Read the model definition and answer for the solid it produces. Units are mm, in the model's axes. Round coordinates to 2 decimals unless told otherwise and drop trailing zeros. Write each loop counter-clockwise with the first axis right and the second up, starting at its lowest first coordinate (ties: lowest second). Pieces come first, ordered by that corner, then holes. Notation, with made-up numbers: (79, -3) -> (103, -3) arc R20 ccw to (103, 33) -> close; hole circle Ø1 at (10, 46.25). An arc over 180 degrees is marked (long way). Return JSON: item names as keys, results as strings.
Solid Edge part; units mm, degrees
sketch "Sketch1" plane through (0, 0, 0) normal (0, -1, 0) x (1, 0, 0)
  line L0 (0, 0) -> (0, -2.95)
  line L1 (0, -2.95) -> (0.3349, -4.2)
  line L2 (0.3349, -4.2) -> (2.8651, -4.2)
  line L3 (2.8651, -4.2) -> (3.2, -2.95)
  line L4 (3.2, -2.95) -> (3.2, 0)
  line L5 (3.2, 0) -> (0, 0)
revolve "RevolvedProtrusion1" add sketch "Sketch1" angle 360 about axis through (3.2, 0, 0) along (-1, 0, 0)
sketch "Sketch2" plane through (0, 0, 0) normal (1, 0, 0) x (0, 1, 0)
  line L0 (14, 14) -> (-14, 14)
  line L1 (-14, 14) -> (-14, -14)
  line L2 (-14, -14) -> (14, -14)
  line L3 (14, -14) -> (14, 14)
  line L4 (2.0207, 3.5) -> (-2.0207, 3.5)
  line L5 (-2.0207, 3.5) -> (-4.0415, 0)
  line L6 (-4.0415, 0) -> (-2.0207, -3.5)
  line L7 (-2.0207, -3.5) -> (2.0207, -3.5)
  line L8 (2.0207, -3.5) -> (4.0415, 0)
  line L9 (4.0415, 0) -> (2.0207, 3.5)
extrude "ExtrudedCutout_1" cut sketch "Sketch2" against normal blind 4.2 and the other way blind 4.2
sketch "Sketch3" plane through (0, 0, 0) normal (0, 0, 1) x (1, 0, 0)
  line L0 (0, 0) -> (0, 2)
  line L1 (0, 2) -> (0.379, 1.621)
  line L2 (0.379, 1.621) -> (2.821, 1.621)
  line L3 (2.821, 1.621) -> (3.2, 2)
  line L4 (3.2, 2) -> (3.2, 0)
  line L5 (3.2, 0) -> (0, 0)
revolve "RevolvedCutout1" cut sketch "Sketch3" angle 360 about axis through (3.2, 0, 0) along (-1, 0, 0)
cosmetic_thread "Thread1"
properties part number "Hexagon nut - style 1 JIS B 1181 M4"
Item 1: Straight lines are drawn through the part: L1, parallel to Z at x = 1.9, y = 0; L2, parallel to Y at x = 0.75, z = 2; L3, parallel to Y at x = 3, z = 1.5. For each, find the intervals that lie inside material, in ascending order. Write a range as [from, to].
Worked answers:
{"L1": "z = [-3.5, -1.62], [1.62, 3.5]", "L2": "y = [-2.89, 2.89]", "L3": "y = [-3.18, -0.99], [0.99, 3.18]"}
Item 2: Section A-A (y = 0) is taken. Give the vertices of the cut face in (x, z), then the cut area to 3 significant figures.
Worked answers:
{"outline": "(0, -2.95) -> (0.15, -3.5) -> (3.05, -3.5) -> (3.2, -2.95) -> (3.2, -2) -> (2.82, -1.62) -> (0.38, -1.62) -> (0, -2) -> close; (0, 2) -> (0.38, 1.62) -> (2.82, 1.62) -> (3.2, 2) -> (3.2, 2.95) -> (3.05, 3.5) -> (0.15, 3.5) -> (0, 2.95) -> close", "area": "11.6 mm2"}
Item 3: For a pull along Z with two mould halves and no side action, classify faces 1 (the flat face through (3.2, 1, -2)), 2 (the flat face through (1.62, 3.045, 1.726)), 3 (the cylindrical face through (1.617, 0.748, -1.438)) as released by +Z, released by -Z, zero draft, split by the parting line, or undercut.
Worked answers:
{"face 1": "zero draft", "face 2": "released by +Z", "face 3": "undercut"}
Item 4: Section B-B (x = 1.5) is taken. Give the vertices of the cut face in (y, z), then the cut area to 3 significant figures.
Worked answers:
{"outline": "(-4.04, 0) -> (-2.02, -3.5) -> (2.02, -3.5) -> (4.04, 0) -> (2.02, 3.5) -> (-2.02, 3.5) -> close; hole circle Ø3.24 at (0, 0)", "area": "34.2 mm2"}
Item 5: A flat-ended cylindrical pin translates along its axis: pin 1 (3 mm diameter, centred on y = 0, z = 0, fed in from +X). Find the tip coordinate at first contact, or state that the pin passes through.
Worked answers:
{"pin 1": "passes through"}
